Build history of the part. All positions in model axes, mm. Face numbers are marked on the shaded views. A direction names the side the tool comes from. Coordinates: 2 decimals unless noted, no trailing zeros. Loops run counter-clockwise (first coordinate to the right, second up) from the corner with the lowest first, then second, coordinate; pieces in that order, holes last. Notation, with made-up numbers: (60, 46) -> (81, 46) arc R26 ccw to (81, 71) -> close; hole circle Ø4 at (46, -33). An arc over 180 degrees is marked (long way). One line per item, written item: value. Start each with the question number.
```python
from build123d import *

# Parameters (mm, degrees)
FILLET1_R = 0.5


with BuildPart() as part:
    # Sketch1 → Revolve1 (revolve)
    with BuildSketch(Plane.XY):
        Polygon((2.5, 0), (3.5, 0), (5, 10.8), (3.4, 10.8), (3.4, 7.8), (2.5, 7.8), align=None)
    revolve(axis=Axis((0, 0, 0), (0, 1, 0)))

    # Fillet1
    fillet1_edges = [part.edges().sort_by_distance(p)[0] for p in [
        (-5, 10.8, 0),
    ]]
    fillet(fillet1_edges, radius=FILLET1_R)


solid = part.part
```
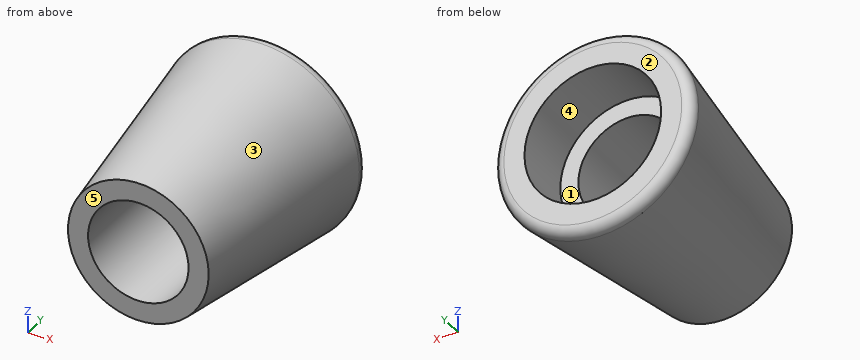
Item 1: Two-plate mould, pull along Z, no slides. Class the marked faces 1, 2 and 3: +Z half, -Z half, draft (parallel to the pull), parting line (faces both ways), or undercut.
Item 2: Band-saw the part on D-D, the plane y = 3.25. List the corners of the cut face in (x, z), and give its area (3 significant figures).
Item 3: Band-saw the part on C-C, the plane y = 5. List the corners of the cut face in (x, z).
Item 4: Band-saw the part on B-B, the plane x = 0. List the corners of the cut face in (y, z).
Item 5: Tool access for the marked faces 4 and 5: list every direction of +Z, -Z, +X, -X, +Y, -Y with a clear straight run to the whole face (end or side of a thin tool).
Item 6: Probe probe 1 along Z at (x, y) = (0, 10.25); probe 2 along X at (y, z) = (9.55, 0); probe 3 along Z at (x, y) = (0, 5.75). List the from-to ranges inside material, lowest first.
Item 7: Drop flat-ended pins along their axis: pin 1 Ø3 at (y, z) = (1.5, -2) entering from -X; pin 2 Ø4 at (x, y) = (-1, 7.5) entering from +Z; pin 3 Ø4 at (x, y) = (-3.5, 6) entering from +Z. Give the stop position or say it passes through.
Item 8: Band-saw the part on A-A, the plane z = 0. List the corners of the cut face in (x, y).
Worked out:
1. face 1: undercut
1. face 2: draft
1. face 3: parting line
2. outline: circle Ø7.9 at (0, 0); hole circle Ø5 at (0, 0)
2. area: 29.4 mm²
3. outline: circle Ø8.39 at (0, 0); hole circle Ø5 at (0, 0)
4. outline: (0, -3.5) -> (10.23, -4.92) arc R0.5 ccw to (10.8, -4.43) -> (10.8, -3.4) -> (7.8, -3.4) -> (7.8, -2.5) -> (0, -2.5) -> close; (0, 2.5) -> (7.8, 2.5) -> (7.8, 3.4) -> (10.8, 3.4) -> (10.8, 4.43) arc R0.5 ccw to (10.23, 4.92) -> (0, 3.5) -> close
5. face 4: +Y
5. face 5: +Z, -Z, +X, -X, -Y
6. probe 1: z = -4.92 to -3.4, 3.4 to 4.92
6. probe 2: x = -4.83 to -3.4, 3.4 to 4.83
6. probe 3: z = -4.3 to -2.5, 2.5 to 4.3
7. pin 1: stops at x = -3.75
7. pin 2: stops at z = 4.79
7. pin 3: stops at z = 4.12
8. outline: (-4.92, 10.23) -> (-3.5, 0) -> (-2.5, 0) -> (-2.5, 7.8) -> (-3.4, 7.8) -> (-3.4, 10.8) -> (-4.43, 10.8) arc R0.5 ccw to start; (2.5, 0) -> (3.5, 0) -> (4.92, 10.23) arc R0.5 ccw to (4.43, 10.8) -> (3.4, 10.8) -> (3.4, 7.8) -> (2.5, 7.8) -> close
